```python
from build123d import *

# Parameters (mm, degrees)
SKETCH1_W                    = 44
SKETCH1_H                    = 37
SKETCH1_R                    = 1.75
BASE_FLANGE1_DEPTH           = 3.175
EDGE_FLANGE1_STRIP_W         = 16.51
EDGE_FLANGE1_STRIP_H         = 3.175
EDGE_FLANGE1_STRIP_CUT_DEPTH = 44
EDGE_FLANGE1_DEPTH           = 44
EDGE_FLANGE2_STRIP_W         = 16.51
EDGE_FLANGE2_STRIP_H         = 3.175
EDGE_FLANGE2_STRIP_CUT_DEPTH = 44
EDGE_FLANGE2_DEPTH           = 44
CUT_EXTRUDE1_REACH           = 69.497
SKETCH12_R                   = 11.25
SKETCH12_R_2                 = 1.6
CUT_EXTRUDE2_REACH           = 69.497
CHAMFER1_SIZE                = 7
FILLET1_R                    = 5
SKETCH14_W                   = 8.7
SKETCH14_H                   = 10
SKETCH14_R                   = 1.6
SKETCH14_W_2                 = 13.3
BOSS_EXTRUDE1_DEPTH          = 3.175
FILLET2_R                    = 5
FILLET3_R                    = 3


# Sheet-metal steps are written as plain solids
with BuildPart() as part:
    # Sketch1 → Base-Flange1 (new body)
    with BuildSketch(Plane(origin=(0, 0, 0), x_dir=(1, 0, 0), z_dir=(0, 1, 0))):
        Rectangle(SKETCH1_W, SKETCH1_H)
        with Locations(Location((-10, 11, 0), (0, 0, 270))):
            Circle(SKETCH1_R, mode=Mode.SUBTRACT)
        with Locations(Location((10, 11, 0), (0, 0, 270))):
            Circle(SKETCH1_R, mode=Mode.SUBTRACT)
        with Locations(Location((10, -9, 0), (0, 0, 270))):
            Circle(SKETCH1_R, mode=Mode.SUBTRACT)
        with Locations(Location((-10, -9, 0), (0, 0, 270))):
            Circle(SKETCH1_R, mode=Mode.SUBTRACT)
    extrude(amount=-BASE_FLANGE1_DEPTH)

    # Edge-Flange1 strip (across the edge) → Edge-Flange1 strip cut (cut)
    with BuildSketch(Plane(origin=(22, 0, -18.5), x_dir=(0, 0, 1), z_dir=(-1, 0, 0))):
        with Locations((-6.35, -1.5875)):
            Rectangle(EDGE_FLANGE1_STRIP_W, EDGE_FLANGE1_STRIP_H)
    extrude(amount=EDGE_FLANGE1_STRIP_CUT_DEPTH, mode=Mode.SUBTRACT)

    # Edge-Flange1 section (across the edge) → Edge-Flange1 (add)
    with BuildSketch(Plane(origin=(22, 0, -18.5), x_dir=(0, 0, 1), z_dir=(-1, 0, 0))):
        with BuildLine():
            Line((-3.175, 1.905), (-3.175, 46.825))
            Line((-3.175, 46.825), (0, 46.825))
            Line((0, 46.825), (0, 1.905))
            ThreePointArc((0, 1.905), (0.557961582, 0.557961582), (1.905, 0))
            Line((1.905, 0), (1.905, -3.175))
            ThreePointArc((1.905, -3.175), (-1.687102448, -1.687102448), (-3.175, 1.905))
        make_face()
    extrude(amount=EDGE_FLANGE1_DEPTH)

    # Edge-Flange2 strip (across the edge) → Edge-Flange2 strip cut (cut)
    with BuildSketch(Plane(origin=(22, -3.175, 18.5), x_dir=(0, 0, -1), z_dir=(-1, 0, 0))):
        with Locations((-6.35, -1.5875)):
            Rectangle(EDGE_FLANGE2_STRIP_W, EDGE_FLANGE2_STRIP_H)
    extrude(amount=EDGE_FLANGE2_STRIP_CUT_DEPTH, mode=Mode.SUBTRACT)

    # Edge-Flange2 section (across the edge) → Edge-Flange2 (add)
    with BuildSketch(Plane(origin=(22, -3.175, 18.5), x_dir=(0, 0, -1), z_dir=(-1, 0, 0))):
        with BuildLine():
            Line((-3.175, 1.905), (-3.175, 16.825))
            Line((-3.175, 16.825), (0, 16.825))
            Line((0, 16.825), (0, 1.905))
            ThreePointArc((0, 1.905), (0.557961582, 0.557961582), (1.905, 0))
            Line((1.905, 0), (1.905, -3.175))
            ThreePointArc((1.905, -3.175), (-1.687102448, -1.687102448), (-3.175, 1.905))
        make_face()
    extrude(amount=EDGE_FLANGE2_DEPTH)

    # Sketch12 → Cut-Extrude1 (cut, up to next)
    with BuildSketch(Plane(origin=(0, 0, -21.675), x_dir=(-1, 0, 0), z_dir=(0, 0, -1)), mode=Mode.PRIVATE) as cut_extrude1_sk1:
        with Locations(Location((0, 25.675, 0), (0, 0, 90))):
            Circle(SKETCH12_R)
    cut_extrude1_tool1 = extrude(cut_extrude1_sk1.sketch, amount=-CUT_EXTRUDE1_REACH, mode=Mode.PRIVATE) & part.part
    # Sketch12 → Cut-Extrude1 (cut, up to next)
    with BuildSketch(Plane(origin=(0, 0, -21.675), x_dir=(-1, 0, 0), z_dir=(0, 0, -1)), mode=Mode.PRIVATE) as cut_extrude1_sk2:
        with Locations(Location((15.5, 41.175, 0), (0, 0, 90))):
            Circle(SKETCH12_R_2)
    cut_extrude1_tool2 = extrude(cut_extrude1_sk2.sketch, amount=-CUT_EXTRUDE1_REACH, mode=Mode.PRIVATE) & part.part
    # Sketch12 → Cut-Extrude1 (cut, up to next)
    with BuildSketch(Plane(origin=(0, 0, -21.675), x_dir=(-1, 0, 0), z_dir=(0, 0, -1)), mode=Mode.PRIVATE) as cut_extrude1_sk3:
        with Locations(Location((15.5, 10.175, 0), (0, 0, 90))):
            Circle(SKETCH12_R_2)
    cut_extrude1_tool3 = extrude(cut_extrude1_sk3.sketch, amount=-CUT_EXTRUDE1_REACH, mode=Mode.PRIVATE) & part.part
    # Sketch12 → Cut-Extrude1 (cut, up to next)
    with BuildSketch(Plane(origin=(0, 0, -21.675), x_dir=(-1, 0, 0), z_dir=(0, 0, -1)), mode=Mode.PRIVATE) as cut_extrude1_sk4:
        with Locations(Location((-15.5, 10.175, 0), (0, 0, 90))):
            Circle(SKETCH12_R_2)
    cut_extrude1_tool4 = extrude(cut_extrude1_sk4.sketch, amount=-CUT_EXTRUDE1_REACH, mode=Mode.PRIVATE) & part.part
    # Sketch12 → Cut-Extrude1 (cut, up to next)
    with BuildSketch(Plane(origin=(0, 0, -21.675), x_dir=(-1, 0, 0), z_dir=(0, 0, -1)), mode=Mode.PRIVATE) as cut_extrude1_sk5:
        with Locations(Location((-15.5, 41.175, 0), (0, 0, 90))):
            Circle(SKETCH12_R_2)
    cut_extrude1_tool5 = extrude(cut_extrude1_sk5.sketch, amount=-CUT_EXTRUDE1_REACH, mode=Mode.PRIVATE) & part.part
    add(cut_extrude1_tool1.solids().sort_by_distance((0, 25.675, -21.675))[0], mode=Mode.SUBTRACT)
    add(cut_extrude1_tool2.solids().sort_by_distance((-15.5, 41.175, -21.675))[0], mode=Mode.SUBTRACT)
    add(cut_extrude1_tool3.solids().sort_by_distance((-15.5, 10.175, -21.675))[0], mode=Mode.SUBTRACT)
    add(cut_extrude1_tool4.solids().sort_by_distance((15.5, 10.175, -21.675))[0], mode=Mode.SUBTRACT)
    add(cut_extrude1_tool5.solids().sort_by_distance((15.5, 41.175, -21.675))[0], mode=Mode.SUBTRACT)

    # Sketch13 → Cut-Extrude2 (cut, up to next)
    with BuildSketch(Plane.XY.offset(21.675), mode=Mode.PRIVATE) as cut_extrude2_sk1:
        with BuildLine():
            Line((-6.75, -12.975), (-6.75, -6.975))
            ThreePointArc((-6.75, -6.975), (-5, -5.225), (-3.25, -6.975))
            Line((-3.25, -6.975), (-3.25, -12.975))
            ThreePointArc((-3.25, -12.975), (-5, -14.725), (-6.75, -12.975))
        make_face()
    cut_extrude2_tool1 = extrude(cut_extrude2_sk1.sketch, amount=-CUT_EXTRUDE2_REACH, mode=Mode.PRIVATE) & part.part
    # Sketch13 → Cut-Extrude2 (cut, up to next)
    with BuildSketch(Plane.XY.offset(21.675), mode=Mode.PRIVATE) as cut_extrude2_sk2:
        with BuildLine():
            Line((-16.75, -12.975), (-16.75, -6.975))
            ThreePointArc((-16.75, -6.975), (-15, -5.225), (-13.25, -6.975))
            Line((-13.25, -6.975), (-13.25, -12.975))
            ThreePointArc((-13.25, -12.975), (-15, -14.725), (-16.75, -12.975))
        make_face()
    cut_extrude2_tool2 = extrude(cut_extrude2_sk2.sketch, amount=-CUT_EXTRUDE2_REACH, mode=Mode.PRIVATE) & part.part
    # Sketch13 → Cut-Extrude2 (cut, up to next)
    with BuildSketch(Plane.XY.offset(21.675), mode=Mode.PRIVATE) as cut_extrude2_sk3:
        with BuildLine():
            Line((16.75, -12.975), (16.75, -6.975))
            ThreePointArc((16.75, -6.975), (15, -5.225), (13.25, -6.975))
            Line((13.25, -6.975), (13.25, -12.975))
            ThreePointArc((13.25, -12.975), (15, -14.725), (16.75, -12.975))
        make_face()
    cut_extrude2_tool3 = extrude(cut_extrude2_sk3.sketch, amount=-CUT_EXTRUDE2_REACH, mode=Mode.PRIVATE) & part.part
    # Sketch13 → Cut-Extrude2 (cut, up to next)
    with BuildSketch(Plane.XY.offset(21.675), mode=Mode.PRIVATE) as cut_extrude2_sk4:
        with BuildLine():
            Line((6.75, -12.975), (6.75, -6.975))
            ThreePointArc((6.75, -6.975), (5, -5.225), (3.25, -6.975))
            Line((3.25, -6.975), (3.25, -12.975))
            ThreePointArc((3.25, -12.975), (5, -14.725), (6.75, -12.975))
        make_face()
    cut_extrude2_tool4 = extrude(cut_extrude2_sk4.sketch, amount=-CUT_EXTRUDE2_REACH, mode=Mode.PRIVATE) & part.part
    add(cut_extrude2_tool1.solids().sort_by_distance((-5, -9.975, 21.675))[0], mode=Mode.SUBTRACT)
    add(cut_extrude2_tool2.solids().sort_by_distance((-15, -9.975, 21.675))[0], mode=Mode.SUBTRACT)
    add(cut_extrude2_tool3.solids().sort_by_distance((15, -9.975, 21.675))[0], mode=Mode.SUBTRACT)
    add(cut_extrude2_tool4.solids().sort_by_distance((5, -9.975, 21.675))[0], mode=Mode.SUBTRACT)

    # Chamfer1
    chamfer1_edges = [part.edges().sort_by_distance(p)[0] for p in [
        (22, -20, 20.0875),
        (-22, -20, 20.0875),
    ]]
    chamfer(chamfer1_edges, length=CHAMFER1_SIZE)

    # Fillet1
    fillet1_edges = [part.edges().sort_by_distance(p)[0] for p in [
        (15, -20, 20.0875),
        (-15, -20, 20.0875),
        (-22, -13, 20.0875),
        (22, -13, 20.0875),
        (22, 46.825, -20.0875),
        (-22, 46.825, -20.0875),
    ]]
    fillet(fillet1_edges, radius=FILLET1_R)

    # Sketch14 → Boss-Extrude1 (add)
    # profile 1 of 2: a face of its own
    with BuildSketch(Plane(origin=(0, 0, -21.675), x_dir=(-1, 0, 0), z_dir=(0, 0, -1))):
        with Locations((-26.35, 10.525)):
            Rectangle(SKETCH14_W, SKETCH14_H)
        with Locations(Location((-25.7, 10.525, 0), (0, 0, 90))):
            Circle(SKETCH14_R, mode=Mode.SUBTRACT)
    # profile 2 of 2: a face of its own
    with BuildSketch(Plane(origin=(0, 0, -21.675), x_dir=(-1, 0, 0), z_dir=(0, 0, -1))):
        with Locations((28.65, 10.525)):
            Rectangle(SKETCH14_W_2, SKETCH14_H)
        with Locations(Location((30.3, 10.525, 0), (0, 0, 90))):
            Circle(SKETCH14_R, mode=Mode.SUBTRACT)
    extrude(amount=-BOSS_EXTRUDE1_DEPTH)

    # Fillet2
    fillet2_edges = [part.edges().sort_by_distance(p)[0] for p in [
        (-22, 15.525, -20.0875),
        (22, 15.525, -20.0875),
    ]]
    fillet(fillet2_edges, radius=FILLET2_R)

    # Fillet3
    fillet3_edges = [part.edges().sort_by_distance(p)[0] for p in [
        (-35.3, 15.525, -20.0875),
        (-35.3, 5.525, -20.0875),
        (30.7, 5.525, -20.0875),
        (30.7, 15.525, -20.0875),
    ]]
    fillet(fillet3_edges, radius=FILLET3_R)


solid = part.part
```
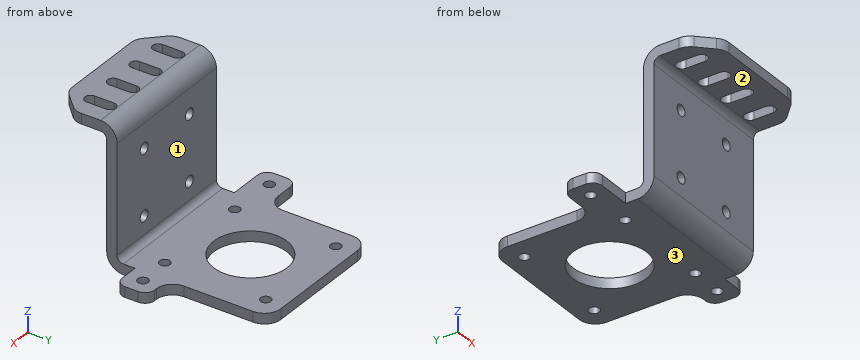
Input: part model. Units: mm. Frame: model coordinates. Face numbers are marked on the shaded views. A direction names the side the tool comes from. Round coordinates to 2 decimals unless told otherwise and drop trailing zeros. Order: outer loops, then holes, each group sorted by start corner. A loop starts at its lowest first (then second) coordinate and runs counter-clockwise, first axis right, second up. Notation, with made-up numbers: (-4, -22.75) - (47, -22.75) arc R22 cw to (47, -6.75) - close; hole circle Ø9 at (62, -1.75). An arc over 180 degrees is marked (long way). One line per question, with ' | ' between items. Start each with the question number.
1) Cut plane B-B, the plane z = -11. Return the cut outline in (x, y) (3 decimals), then the cut area to 3 significant figures.
2) Ray query, probe 1 along X at (y, z) = (-2.45, -11); probe 2 along Y at (x, z) = (-8, 10) (3 decimals); probe 3 along Z at (x, y) = (12, -10.5) (3 decimals). Return the intervals inside material, ascending.
3) Set-up query: the marked faces 1, 2 and 3. Return all of +Z, -Z, +X, -X, +Y, -Y with unobstructed straight access to the full face (end or side cutting, diameter ignored); none if empty.
4) Cut plane C-C, the plane y = 22. Return the cut outline in (x, z) (3 decimals), then the cut area to 3 significant figures.
5) Cut plane D-D, the plane x = -4.5. Return the cut outline in (y, z) (3 decimals), then the cut area to 3 significant figures.
6) Cut plane A-A, the plane x = -30.3. Return the cut outline in (y, z) (3 decimals).
7) Contact query for flat-ended pins moving along their axis: P1, Ø4, axis at x = 5, z = -15.5, coming from the -Y side (3 decimals); P2, Ø3, axis at y = -2.5, z = 4, coming from the -X side; P3, Ø12, axis at x = -3, z = 3, coming from the +Y side; P4, Ø3.5, axis at x = 15.5, y = 41.175, coming from the -Z side (3 decimals). Output: stop coordinate, or through.
Worked out:
1) outline: (-22, -3.175) - (-11.75, -3.175) - (-11.75, 0) - (-22, 0) - close; (-8.25, -3.175) - (8.25, -3.175) - (8.25, 0) - (-8.25, 0) - close; (11.75, -3.175) - (22, -3.175) - (22, 0) - (11.75, 0) - close | area: 117 mm^2
2) probe 1: x = -22 to -11.75, -8.25 to 8.25, 11.75 to 22 | probe 2: y = -3.175 to 0 | probe 3: z = 18.5 to 21.675
3) face 1: +Z, +X, -X, +Y | face 2: -Z, +X, -X, -Y | face 3: -Z, +X, -X, +Y, -Y
4) outline: (-22, -21.675) - (-10.633, -21.675) - (-10.633, -18.5) - (-22, -18.5) - close; (10.633, -21.675) - (22, -21.675) - (22, -18.5) - (10.633, -18.5) - close | area: 72.2 mm^2
5) outline: (-20, 18.5) - (-14.652, 18.5) - (-14.652, 21.675) - (-20, 21.675) - close; (-5.298, 18.5) - (-5.08, 18.5) arc R1.905 cw to (-3.175, 16.595) - (-3.175, -16.595) arc R5.08 ccw to (1.905, -21.675) - (15.364, -21.675) - (15.364, -18.5) - (1.905, -18.5) arc R1.905 cw to (0, -16.595) - (0, 16.595) arc R5.08 ccw to (-5.08, 21.675) - (-5.298, 21.675) - close; (35.986, -21.675) - (46.825, -21.675) - (46.825, -18.5) - (35.986, -18.5) - close | area: 235 mm^2
6) outline: (5.525, -21.675) - (8.925, -21.675) - (8.925, -18.5) - (5.525, -18.5) - close; (12.125, -21.675) - (15.525, -21.675) - (15.525, -18.5) - (12.125, -18.5) - close
7) P1: stops at y = -3.175 | P2: stops at x = -22 | P3: stops at y = 0 | P4: stops at z = -21.675
